For this review, take the finished solid that the model builds, in its own axes (mm). A direction names the side the tool comes from. Give positions to 0.01 mm unless a question says otherwise; leave off trailing zeros. Order: outer loops, then holes, each group sorted by start corner. A loop starts at its lowest first (then second) coordinate and runs counter-clockwise, first axis right, second up. Notation, with made-up numbers: (39, 22.5) - (63, 22.5) arc R11 ccw to (63, 35.5) - close; hole circle Ø4 at (60, 17). An arc over 180 degrees is marked (long way). Answer as a JSON object with one key per item and string values. Group by question number.
from build123d import *

# Parameters (mm, degrees)
BOSS_EXTRUDE1_DEPTH = 2
SKETCH3_W           = 7.5
SKETCH3_H           = 7.5
BOSS_EXTRUDE2_DEPTH = 30
BOSS_EXTRUDE3_DEPTH = 2


with BuildPart() as part:
    # Sketch2 → Boss-Extrude1 (new body)
    with BuildSketch(Plane(origin=(0, 0, 0), x_dir=(1, 0, 0), z_dir=(0, 1, 0))):
        Polygon((0, 35), (0, -35), (-22.5, -35), (-22.5, -85), (12.5, -85), (12.5, -60), (100, -75), (150, -75), (150, 75), (100.180900235, 75), (12.680900235, 60), (12.5, 60), (12.5, 85), (-22.5, 85), (-22.5, 35), align=None)
    extrude(amount=BOSS_EXTRUDE1_DEPTH)

    # Sketch3 → Boss-Extrude2 (add)
    with BuildSketch(Plane(origin=(0, 2, 0), x_dir=(1, 0, 0), z_dir=(0, 1, 0))):
        with Locations((146.25, 71.25)):
            Rectangle(SKETCH3_W, SKETCH3_H)
        with Locations((146.25, -71.25)):
            Rectangle(SKETCH3_W, SKETCH3_H)
        with Locations((-18.75, 81.25)):
            Rectangle(SKETCH3_W, SKETCH3_H)
        with Locations((-18.75, -81.25)):
            Rectangle(SKETCH3_W, SKETCH3_H)
    extrude(amount=BOSS_EXTRUDE2_DEPTH)

    # Sketch5 → Boss-Extrude3 (add)
    with BuildSketch(Plane(origin=(0, 32, 0), x_dir=(1, 0, 0), z_dir=(0, 1, 0))):
        Polygon((150, 75), (100, 75), (12.5, 60), (12.5, 85), (-22.5, 85), (-22.5, 65), (-22.5, 35), (39.717843368, 35), (39.717843368, -35), (-22.5, -35), (-22.5, -85), (12.5, -85), (12.5, -60), (100, -75), (150, -75), align=None)
    extrude(amount=BOSS_EXTRUDE3_DEPTH)


solid = part.part
1) Consider section A-A (x = 124). Give the boundary of the cut face in (y, z).
2) Consider section B-B (y = 17). Give the boundary of the cut face in (x, z).
3) Consider section C-C (z = 16.5). Give the boundary of the cut face in (x, y), plus the area to 3 significant figures.
4) For pin 1 (8 mm diameter, centred on x = 146.5, y = 23.5, fed in from +Z); pin 2 (1.6 mm diameter, centred on y = 1.5, z = 75.5, fed in from +X); pin 3 (2 mm diameter, centred on y = 23, z = 80, fed in from +X); pin 4 (8 mm diameter, centred on x = 146.5, y = 19.5, fed in from -Z), all flat-tipped, find the tip position at first contact; note any pin that passes through.
5) Mouldability with a two-part tool opening along X and no side actions: class faces 4 (the face through (56.862, 32.986, -67.605)), 5 (the face through (143, 17, 75)), 6 (the face through (-22.5, 17, 78)) as released by +X, released by -X, zero draft, split by the parting line, or undercut.
6) For line 1 (Y direction, x = 86, z = -62.5); line 2 (Y direction, x = 8.5, z = -34); line 3 (X direction, y = 19, z = 71), list the stretches that pass through material, from the lowest coordinate up.
7) For faces 1 (the face through (144, 18, -75)), 2 (the face through (-15, 17, -81)), 3 (the face through (146, 17, -67.5)), list the 3-axis set-ups (+Z, -Z, +X, -X, +Y, -Y) from which the entire face can be reached by the end or side of a thin tool; tool diameter is ignored.
8) Consider section D-D (x = -11). Give the boundary of the cut face in (y, z).
Result set:
{
 "1": {"outline": "(0, -75) - (2, -75) - (2, 75) - (0, 75) - close; (32, -75) - (34, -75) - (34, 75) - (32, 75) - close"},
 "2": {"outline": "(-22.5, -85) - (-15, -85) - (-15, -77.5) - (-22.5, -77.5) - close; (-22.5, 77.5) - (-15, 77.5) - (-15, 85) - (-22.5, 85) - close; (142.5, -75) - (150, -75) - (150, -67.5) - (142.5, -67.5) - close; (142.5, 67.5) - (150, 67.5) - (150, 75) - (142.5, 75) - close"},
 "3": {"outline": "(0, 0) - (150, 0) - (150, 2) - (0, 2) - close; (39.72, 32) - (150, 32) - (150, 34) - (39.72, 34) - close", "area": "521 mm2"},
 "4": {"pin 1": "stops at z = 75", "pin 2": "stops at x = 150", "pin 3": "stops at x = -15", "pin 4": "stops at z = -75"},
 "5": {"face 4": "undercut", "face 5": "zero draft", "face 6": "released by -X"},
 "6": {"line 1": "y = 0 to 2, 32 to 34", "line 2": "y = 0 to 2", "line 3": "x = 142.5 to 150"},
 "7": {"face 1": "-Z, +X, +Y, -Y", "face 2": "+Z, -Z, +X", "face 3": "+X, -X"},
 "8": {"outline": "(0, -85) - (2, -85) - (2, -35) - (0, -35) - close; (0, 35) - (2, 35) - (2, 85) - (0, 85) - close; (32, -85) - (34, -85) - (34, -35) - (32, -35) - close; (32, 35) - (34, 35) - (34, 85) - (32, 85) - close"}
}
